from build123d import *

# Parameters (mm, degrees)
SKETCH1_R           = 2
BOSS_EXTRUDE1_DEPTH = 3.2
SKETCH2_OUTSIDE_W   = 19.632
SKETCH2_OUTSIDE_H   = 20.714
SKETCH2_OUTSIDE_R   = 3.5
CUT_EXTRUDE1_DEPTH  = 4.2
CUT_EXTRUDE1_TAPER  = 45
SKETCH3_OUTSIDE_W   = 19.632
SKETCH3_OUTSIDE_H   = 20.714
SKETCH3_OUTSIDE_R   = 3.5
CUT_EXTRUDE2_DEPTH  = 4.2
CUT_EXTRUDE2_TAPER  = 45


with BuildPart() as part:
    # Sketch1 → Boss-Extrude1 (new body)
    with BuildSketch(Plane(origin=(0, 0, 0), x_dir=(1, 0, 0), z_dir=(0, 1, 0))):
        Polygon((0, 4.041451884), (-3.5, 2.020725942), (-3.5, -2.020725942), (0, -4.041451884), (3.5, -2.020725942), (3.5, 2.020725942), align=None)
        Circle(SKETCH1_R, mode=Mode.SUBTRACT)
    extrude(amount=BOSS_EXTRUDE1_DEPTH)

    # Sketch2 outside → Cut-Extrude1 (cut, through all)
    with BuildSketch(Plane(origin=(0, 3.2, 0), x_dir=(1, 0, 0), z_dir=(0, 1, 0))):
        Rectangle(SKETCH2_OUTSIDE_W, SKETCH2_OUTSIDE_H)
        Circle(SKETCH2_OUTSIDE_R, mode=Mode.SUBTRACT)
    extrude(amount=-CUT_EXTRUDE1_DEPTH, taper=CUT_EXTRUDE1_TAPER, mode=Mode.SUBTRACT)

    # Sketch3 outside → Cut-Extrude2 (cut, through all)
    with BuildSketch(Plane.XZ):
        Rectangle(SKETCH3_OUTSIDE_W, SKETCH3_OUTSIDE_H)
        Circle(SKETCH3_OUTSIDE_R, mode=Mode.SUBTRACT)
    extrude(amount=-CUT_EXTRUDE2_DEPTH, taper=CUT_EXTRUDE2_TAPER, mode=Mode.SUBTRACT)


solid = part.part
Read the model definition and answer for the solid it produces. Units are mm, in the model's axes. Round coordinates to 2 decimals unless told otherwise and drop trailing zeros. Write each loop counter-clockwise with the first axis right and the second up, starting at its lowest first coordinate (ties: lowest second). Pieces come first, ordered by that corner, then holes.
Q1. Straight lines are drawn through the part: line 1 (X direction, y = 1.6, z = 0); line 2 (Z direction, x = 0.75, y = 1); line 3 (Z direction, x = -1, y = 0.6). For each, find the intervals that lie inside material, in ascending order.
Values:
line 1: x = -3.5 to -2, 2 to 3.5
line 2: z = -3.61 to -1.85, 1.85 to 3.61
line 3: z = -3.46 to -1.73, 1.73 to 3.46
Q2. Flat-ended cylindrical pins translate along their axes: P1, Ø1.5, axis at y = 0.5, z = -3, coming from the +X side; P2, Ø1, axis at x = 1, y = 0.5, coming from the -Z side. Find the tip coordinate at first contact, or state that the pin passes through.
Values:
P1: stops at x = 3.1
P2: stops at z = -3.75
Q3. The mould has two halves that part along X. Classify faces 1 (the face through (0, 2, 2)), 2 (the face through (2, 3.2, 2)), 3 (the face through (3.149, 0.132, -1.808)): released by +X, released by -X, zero draft, split by the parting line, or undercut.
Values:
face 1: undercut
face 2: zero draft
face 3: released by +X
Q4. Find section A-A on y = 2. Determine the outline of the cut face in (x, z).
Values:
outline: (-3.5, -2.02) - (0, -4.04) - (3.5, -2.02) - (3.5, 2.02) - (0, 4.04) - (-3.5, 2.02) - close; hole circle Ø4 at (0, 0)
